The listing builds one solid part. Answer for the finished solid, in the listing's coordinates (mm). A direction names the side the tool comes from. Coordinates: 2 decimals unless noted, no trailing zeros. Write each loop counter-clockwise with the first axis right and the second up, starting at its lowest first coordinate (ties: lowest second). Pieces come first, ordered by that corner, then holes.
from build123d import *

# Parameters (mm, degrees)
SKETCH_W  = 175
SKETCH_H  = 175
SKETCH_R  = 1.6
PAD_DEPTH = 44
FILLET_R  = 5


with BuildPart() as part:
    # Sketch → Pad (new body)
    with BuildSketch(Plane.XY):
        Rectangle(SKETCH_W, SKETCH_H)
        with Locations((-80, 80)):
            Circle(SKETCH_R, mode=Mode.SUBTRACT)
        with Locations((80, 80)):
            Circle(SKETCH_R, mode=Mode.SUBTRACT)
        with Locations((80, -80)):
            Circle(SKETCH_R, mode=Mode.SUBTRACT)
        with Locations((-80, -80)):
            Circle(SKETCH_R, mode=Mode.SUBTRACT)
        with BuildLine():
            Line((-85, 55), (-85, -55))
            ThreePointArc((-85, -55), (-76.213203, -76.213203), (-55, -85))
            Line((-55, -85), (55, -85))
            ThreePointArc((55, -85), (76.213203, -76.213203), (85, -55))
            Line((85, -55), (85, 55))
            ThreePointArc((85, 55), (76.213203, 76.213203), (55, 85))
            Line((55, 85), (-55, 85))
            ThreePointArc((-55, 85), (-76.213203, 76.213203), (-85, 55))
        make_face(mode=Mode.SUBTRACT)
    extrude(amount=PAD_DEPTH)

    # Fillet
    fillet_edges = [part.edges().sort_by_distance(p)[0] for p in [
        (87.5, 87.5, 22),
        (87.5, -87.5, 22),
        (-87.5, -87.5, 22),
        (-87.5, 87.5, 22),
    ]]
    fillet(fillet_edges, radius=FILLET_R)


solid = part.part
1. Section A-A on x = -8.5 is taken. Give the vertices of the cut face in (y, z), then the cut area to 3 significant figures.
Results found:
outline: (-87.5, 0) - (-85, 0) - (-85, 44) - (-87.5, 44) - close; (85, 0) - (87.5, 0) - (87.5, 44) - (85, 44) - close
area: 220 mm2
2. Section C-C on z = 15 is taken. Give the vertices of the cut face in (x, y).
Results found:
outline: (-87.5, -82.5) arc R5 ccw to (-82.5, -87.5) - (82.5, -87.5) arc R5 ccw to (87.5, -82.5) - (87.5, 82.5) arc R5 ccw to (82.5, 87.5) - (-82.5, 87.5) arc R5 ccw to (-87.5, 82.5) - close; hole (-85, -55) arc R30 ccw to (-55, -85) - (55, -85) arc R30 ccw to (85, -55) - (85, 55) arc R30 ccw to (55, 85) - (-55, 85) arc R30 ccw to (-85, 55) - close; hole circle Ø3.2 at (-80, -80); hole circle Ø3.2 at (-80, 80); hole circle Ø3.2 at (80, -80); hole circle Ø3.2 at (80, 80)
3. A tool of negligible diameter and unlimited length cuts with its end or side. For faces 1 (the flat face through (-85, 1, 22)), 2 (the cylindrical face through (86, 86.07, 22.31)), from which of +Z, -Z, +X, -X, +Y, -Y can it reach the whole face along a straight path? Write none if from no direction.
Results found:
face 1: +Z, -Z
face 2: +Z, -Z, +X, +Y
4. For a pull along X with two mould halves and no side action, classify faces 3 (the flat face through (85, -1, 22)), 4 (the cylindrical face through (86, -86.07, 22.31)), 5 (the flat face through (-65, -84, 0)), 6 (the cylindrical face through (-76.445, -75.979, 21.692)) as pulls with the +X half, pulls with the -X half, needs draft (parallel to the pull), parting line crosses it, or undercut.
Results found:
face 3: undercut
face 4: pulls with the +X half
face 5: needs draft
face 6: undercut
5. Find the intervals of material crossed by L1, parallel to X at y = -49.5, z = 25.5; L2, parallel to Y at x = -80, z = 29, in increasing order.
Results found:
L1: x = -87.5 to -85, 85 to 87.5
L2: y = -87.5 to -81.6, -78.4 to -71.58, 71.58 to 78.4, 81.6 to 87.5
